from build123d import *

# Parameters (mm, degrees)
EXTRUDE_1_DEPTH     = 5
CUT_EXTRUDE_1_REACH = 7
EXTRUDE_2_DEPTH     = 5
CUT_EXTRUDE_2_REACH = 7
SKETCH_4_W          = 9.6
SKETCH_4_H          = 50
CUT_EXTRUDE_3_REACH = 7
SKETCH_5_W          = 8
SKETCH_5_H          = 5


with BuildPart() as part:
    # 草图1 → 凸台-拉伸1 (new body)
    with BuildSketch(Plane.XY):
        Polygon((-216, 0), (-216, 10), (-196, 10), (-196, 15), (-146.925227119, 100), (146.925227119, 100), (196, 15), (196, 10), (216, 10), (216, 0), (136, 0), (136, 50), (-136, 50), (-136, 0), align=None)
    extrude(amount=EXTRUDE_1_DEPTH)

    # 草图2 → 切除-拉伸1 (cut, up to next)
    with BuildSketch(Plane.XY.offset(5), mode=Mode.PRIVATE) as cut_extrude_1_sk1:
        with BuildLine():
            Line((-146.925227119, 100), (-126.925227119, 100))
            ThreePointArc((-126.925227119, 100), (-144.245735195, 95.358983849), (-156.925227119, 82.679491924))
            Line((-156.925227119, 82.679491924), (-146.925227119, 100))
        make_face()
    cut_extrude_1_tool1 = extrude(cut_extrude_1_sk1.sketch, amount=-CUT_EXTRUDE_1_REACH, mode=Mode.PRIVATE) & part.part
    add(cut_extrude_1_tool1.solids().sort_by_distance((-144.827064, 96.365874, 5))[0], mode=Mode.SUBTRACT)
    # 草图2 → 切除-拉伸1 (cut, up to next)
    with BuildSketch(Plane.XY.offset(5), mode=Mode.PRIVATE) as cut_extrude_1_sk2:
        with BuildLine():
            Line((146.925227119, 100), (156.925227119, 82.679491924))
            ThreePointArc((156.925227119, 82.679491924), (144.245735195, 95.358983849), (126.925227119, 100))
            Line((126.925227119, 100), (146.925227119, 100))
        make_face()
    cut_extrude_1_tool2 = extrude(cut_extrude_1_sk2.sketch, amount=-CUT_EXTRUDE_1_REACH, mode=Mode.PRIVATE) & part.part
    add(cut_extrude_1_tool2.solids().sort_by_distance((144.827064, 96.365874, 5))[0], mode=Mode.SUBTRACT)

    # 草图3 → 凸台-拉伸2 (add)
    with BuildSketch(Plane.XY.offset(5)):
        with BuildLine():
            Line((-116, 50), (-136, 50))
            Line((-136, 50), (-136, 30))
            ThreePointArc((-136, 30), (-130.142135624, 44.142135624), (-116, 50))
        make_face()
        with BuildLine():
            Line((136, 50), (136, 30))
            ThreePointArc((136, 30), (130.142135624, 44.142135624), (116, 50))
            Line((116, 50), (136, 50))
        make_face()
    extrude(amount=-EXTRUDE_2_DEPTH)

    # 草图4 → 切除-拉伸2 (cut, up to next)
    with BuildSketch(Plane.XY.offset(5), mode=Mode.PRIVATE) as cut_extrude_2_sk1:
        with Locations((0, 50)):
            Rectangle(SKETCH_4_W, SKETCH_4_H)
    cut_extrude_2_tool1 = extrude(cut_extrude_2_sk1.sketch, amount=-CUT_EXTRUDE_2_REACH, mode=Mode.PRIVATE) & part.part
    add(cut_extrude_2_tool1.solids().sort_by_distance((0, 50, 5))[0], mode=Mode.SUBTRACT)

    # 草图5 → 切除-拉伸3 (cut, up to next)
    with BuildSketch(Plane.XY.offset(5), mode=Mode.PRIVATE) as cut_extrude_3_sk1:
        with Locations((-182, 17.5)):
            Rectangle(SKETCH_5_W, SKETCH_5_H)
    cut_extrude_3_tool1 = extrude(cut_extrude_3_sk1.sketch, amount=-CUT_EXTRUDE_3_REACH, mode=Mode.PRIVATE) & part.part
    add(cut_extrude_3_tool1.solids().sort_by_distance((-182, 17.5, 5))[0], mode=Mode.SUBTRACT)
    # 草图5 → 切除-拉伸3 (cut, up to next)
    with BuildSketch(Plane.XY.offset(5), mode=Mode.PRIVATE) as cut_extrude_3_sk2:
        with Locations((-164, 17.5)):
            Rectangle(SKETCH_5_W, SKETCH_5_H)
    cut_extrude_3_tool2 = extrude(cut_extrude_3_sk2.sketch, amount=-CUT_EXTRUDE_3_REACH, mode=Mode.PRIVATE) & part.part
    add(cut_extrude_3_tool2.solids().sort_by_distance((-164, 17.5, 5))[0], mode=Mode.SUBTRACT)
    # 草图5 → 切除-拉伸3 (cut, up to next)
    with BuildSketch(Plane.XY.offset(5), mode=Mode.PRIVATE) as cut_extrude_3_sk3:
        with Locations((164, 17.5)):
            Rectangle(SKETCH_5_W, SKETCH_5_H)
    cut_extrude_3_tool3 = extrude(cut_extrude_3_sk3.sketch, amount=-CUT_EXTRUDE_3_REACH, mode=Mode.PRIVATE) & part.part
    add(cut_extrude_3_tool3.solids().sort_by_distance((164, 17.5, 5))[0], mode=Mode.SUBTRACT)
    # 草图5 → 切除-拉伸3 (cut, up to next)
    with BuildSketch(Plane.XY.offset(5), mode=Mode.PRIVATE) as cut_extrude_3_sk4:
        with Locations((182, 17.5)):
            Rectangle(SKETCH_5_W, SKETCH_5_H)
    cut_extrude_3_tool4 = extrude(cut_extrude_3_sk4.sketch, amount=-CUT_EXTRUDE_3_REACH, mode=Mode.PRIVATE) & part.part
    add(cut_extrude_3_tool4.solids().sort_by_distance((182, 17.5, 5))[0], mode=Mode.SUBTRACT)


solid = part.part
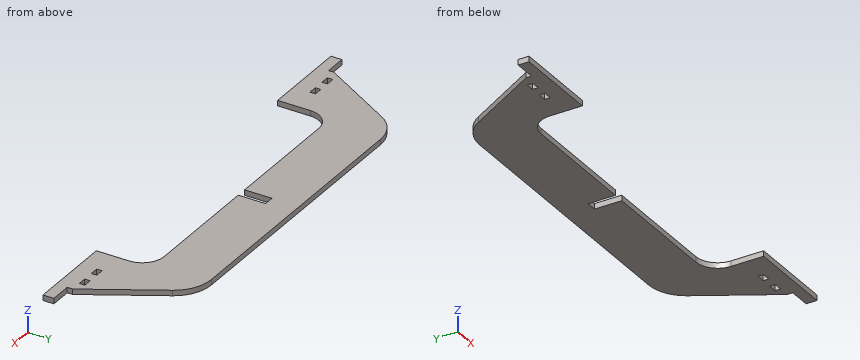
Part model, mm, in its own coordinate system. Round coordinates to 2 decimals unless told otherwise and drop trailing zeros. Write each loop counter-clockwise with the first axis right and the second up, starting at its lowest first coordinate (ties: lowest second). Pieces come first, ordered by that corner, then holes. Notation, with made-up numbers: M 69.5,63 L 127.5,63 A19 ccw 127.5,96 Z; hole C -21,33 d3. An arc over 180 degrees is marked long. Return JSON: item names as keys, results as strings. Group by question number.
(1) Saw through at D-D on x = 62. Write the cut outline in (y, z).
(2) Saw through at A-A on y = 39.5. Write the cut outline in (x, z).
(3) Saw through at C-C on y = 57. Write the cut outline in (x, z), then the cut area to 3 significant figures.
(4) Drill centre lines: probe 1 along X at (y, z) = (16.5, 4.5); probe 2 along Y at (x, z) = (104, 0.85); probe 3 along X at (y, z) = (57.5, 3.7). Where is each one in solid material? Low to high.
(5) Pin check, flat tips, straight feed: pin 1 Ø1.5 at (x, z) = (74, 3) entering from -Y; pin 2 Ø1 at (y, z) = (39.5, 4) entering from -X; pin 3 Ø1.5 at (y, z) = (17, 2.5) entering from -X. Stop position of each tip, or through.
(6) Saw through at B-B on z = 4.05. Count the separate pieces of the cut face and the enclosed holes in it, then the cut area to 3 significant figures.
Returned:
{
 "1": {"outline": "M 50,0 L 100,0 L 100,5 L 50,5 Z"},
 "2": {"outline": "M -181.85,0 L -133.6,0 L -133.6,5 L -181.85,5 Z; M 133.6,0 L 181.85,0 L 181.85,5 L 133.6,5 Z"},
 "3": {"outline": "M -171.75,0 L -4.8,0 L -4.8,5 L -171.75,5 Z; M 4.8,0 L 171.75,0 L 171.75,5 L 4.8,5 Z", "area": "1,670 mm²"},
 "4": {"probe 1": "-195.13 to -186, -178 to -168, -160 to -136, 136 to 160, 168 to 178, 186 to 195.13", "probe 2": "50 to 100", "probe 3": "-171.46 to -4.8, 4.8 to 171.46"},
 "5": {"pin 1": "y = 50", "pin 2": "x = -182.14", "pin 3": "x = -195.28"},
 "6": {"separate pieces": "1", "enclosed holes": "4", "area": "21,500 mm²"}
}
